Source: CAD feature listing. Evaluate the final solid. Frame: model axes, mm. A direction names the side the tool comes from. Give positions to 0.01 mm unless a question says otherwise; leave off trailing zeros. Loops run counter-clockwise (first coordinate to the right, second up) from the corner with the lowest first, then second, coordinate; pieces in that order, holes last. Notation, with made-up numbers: M -17.75,-0.5 L 32.25,-0.5 A11 ccw 32.25,13.5 Z; hole C 35.25,67.25 d7. An arc over 180 degrees is marked long. Answer in a Markdown table with one row per item.
```python
from build123d import *

# Parameters (mm, degrees)
F0_W     = 243.986786
F0_H     = 218.229026
F1_DEPTH = 25.4
F2_R     = 21.192457
F3_DEPTH = 35.958676
F4_R     = 21.528867
F5_DEPTH = 36.293864
F6_R     = 22.840136
F7_DEPTH = 25.4


with BuildPart() as f1:
    # F0 (on Front) → F1 (new body)
    with BuildSketch(Plane.XZ):
        Rectangle(F0_W, F0_H)
    extrude(amount=F1_DEPTH)

    # F2 (on face) → F3 (join)
    with BuildSketch(Plane.XZ.offset(25.4)):
        Circle(F2_R)
    extrude(amount=F3_DEPTH)

    # F4 (on face) → F5 (join)
    with BuildSketch(Plane.XZ.offset(25.4)):
        with Locations((0, 75.056374)):
            Circle(F4_R)
    extrude(amount=F5_DEPTH)

    # F6 (on face) → F7 (join)
    with BuildSketch(Plane.XZ.offset(25.4)):
        with Locations((81.895486, 0)):
            Circle(F6_R)
    extrude(amount=F7_DEPTH)


solid = f1.part
```
Q1. Section query B-B (x = 0). Output: boundary loops of the cut face in (y, z), plus the area to 3 significant figures.
Values follow:
| item | result |
|---|---|
| outline | M -61.69,53.53 L -25.4,53.53 L -25.4,21.19 L -61.36,21.19 L -61.36,-21.19 L -25.4,-21.19 L -25.4,-109.11 L 0,-109.11 L 0,109.11 L -25.4,109.11 L -25.4,96.59 L -61.69,96.59 Z |
| area | 8,630 mm^2 |
Q2. Mould query, pull axis Z, two halves, no side actions, for faces 1 (the flat face through (-2, -13, -109.115)), 2 (the cylindrical face through (-4.59, -43.13, -20.69)), 3 (the cylindrical face through (103.68, -37.92, 6.86)), 4 (the flat face through (-121.993, -13, -2)). Classes: +Z half, -Z half, draft (parallel to the pull), parting line (faces both ways), or undercut.
Values follow:
| item | result |
|---|---|
| face 1 | -Z half |
| face 2 | undercut |
| face 3 | parting line |
| face 4 | draft |
Q3. Reachability of faces 5 (the cylindrical face through (-2.803, -43.293, 96.402)), 6 (the flat face through (0, -61.359, 0)), 7 (the flat face through (82, -50.8, 0)) from +Z, -Z, +X, -X, +Y, -Y: full face, straight path, thin tool, end or side. Return the list, or none.
Values follow:
| item | result |
|---|---|
| face 5 | -Y |
| face 6 | -Z, +X, -X, -Y |
| face 7 | +Z, -Z, +X, -Y |
Q4. Section query C-C (y = -53.5). Output: boundary loops of the cut face in (x, z).
Values follow:
| item | result |
|---|---|
| outline | C 0,75.06 d43.06; C 0,0 d42.38 |
Q5. Section query D-D (x = -104). Output: boundary loops of the cut face in (y, z), plus the area to 3 significant figures.
Values follow:
| item | result |
|---|---|
| outline | M -25.4,-109.11 L 0,-109.11 L 0,109.11 L -25.4,109.11 Z |
| area | 5,540 mm^2 |
Q6. Contact query for flat-ended pins moving along their axis: pin 1 Ø21 at (x, z) = (6, -7.5) entering from -Y; pin 2 Ø3 at (x, z) = (-7.5, 35.5) entering from -Y; pin 3 Ø23 at (x, z) = (88, 4.5) entering from -Y. Output: stop coordinate, or through.
Values follow:
| item | result |
|---|---|
| pin 1 | y = -61.36 |
| pin 2 | y = -25.4 |
| pin 3 | y = -50.8 |
Q7. Section query A-A (z = 0). Output: boundary loops of the cut face in (x, y), plus the area to 3 significant figures.
Values follow:
| item | result |
|---|---|
| outline | M -121.99,-25.4 L -21.19,-25.4 L -21.19,-61.36 L 21.19,-61.36 L 21.19,-25.4 L 59.06,-25.4 L 59.06,-50.8 L 104.74,-50.8 L 104.74,-25.4 L 121.99,-25.4 L 121.99,0 L -121.99,0 Z |
| area | 8,880 mm^2 |
Q8. Ray query, probe 1 along Y at (x, z) = (-34.5, 43); probe 2 along Y at (x, z) = (69, -14); probe 3 along X at (y, z) = (-32.5, 4.5). Return the intervals inside material, ascending. Write a range as from..to.
Values follow:
| item | result |
|---|---|
| probe 1 | -25.4..0 |
| probe 2 | -50.8..0 |
| probe 3 | -20.71..20.71, 59.5..104.29 |
